Could you check a few things on this model? Use its own coordinates, in mm. Face numbers are marked on the shaded views. Coordinates: 2 decimals unless noted, no trailing zeros. Write each loop counter-clockwise with the first axis right and the second up, starting at its lowest first coordinate (ties: lowest second). Pieces come first, ordered by that corner, then holes. Notation, with made-up numbers: M 78,6.5 L 87,6.5 A34 cw 87,44.5 Z; hole C -21,64.5 d7. An arc over 180 degrees is marked long. Answer as CSV lines item,"result". Start each with the question number.
Item 1: Suppose I cut it at D-D, the plane z = -12.25. Write out the boundary of the cut face in (x, y).
Item 2: Suppose I cut it at B-B, the plane z = -6. Write out the boundary of the cut face in (x, y).
Item 3: If I drill on line 1 along X through (y, z) = (5.5, -7.5); line 2 along X through (y, z) = (22.5, -9); line 3 along Z through (x, y) = (-32, 19), over which ranges is the centre line in solid material (lowest first)? Write a range as [from, to].
Item 4: Suppose I cut it at A-A, the plane y = 7. Write out the boundary of the cut face in (x, z).
Item 5: Suppose I cut it at C-C, the plane x = 12.75. Write out the boundary of the cut face in (y, z), and give its area (3 significant figures).
Item 6: We'd pull the mould along X, two halves only. Please class the marked faces 1, 2, 3 and 4: +X half, -X half, draft (parallel to the pull), parting line (faces both ways), or undercut.
Item 7: I'm going to push flat-ended pins straight in: P1, Ø8, axis at x = 14, y = 15.5, coming from the +Z side; P2, Ø5, axis at x = 10.5, y = 25.5, coming from the -Z side. Where does each tip first touch, or does it pass through?
```python
from build123d import *

# Parameters (mm, degrees)
BOSS_EXTRUDE1_DEPTH = 42
FILLET1_R           = 4
SKETCH2_R           = 4
CUT_EXTRUDE1_DEPTH  = 42
SKETCH3_R           = 2
CUT_EXTRUDE2_DEPTH  = 42


with BuildPart() as part:
    # Sketch1 → Boss-Extrude1 (new body)
    with BuildSketch(Plane(origin=(0, 0, 0), x_dir=(1, 0, 0), z_dir=(0, 1, 0))):
        with BuildLine():
            Line((-37.647058824, 19.411764706), (-42.352941176, 10.588235294))
            ThreePointArc((-42.352941176, 10.588235294), (0, 0), (42.352941176, 10.588235294))
            Line((42.352941176, 10.588235294), (37.647058824, 19.411764706))
            ThreePointArc((37.647058824, 19.411764706), (0, 10), (-37.647058824, 19.411764706))
        make_face()
    extrude(amount=BOSS_EXTRUDE1_DEPTH)

    # Fillet1
    fillet1_edges = [part.edges().sort_by_distance(p)[0] for p in [
        (37.647058824, 21, -19.411764706),
        (42.352941176, 21, -10.588235294),
        (-42.352941176, 21, -10.588235294),
        (-37.647058824, 21, -19.411764706),
    ]]
    fillet(fillet1_edges, radius=FILLET1_R)

    # Sketch2 → Cut-Extrude1 (cut)
    with BuildSketch(Plane(origin=(0, 42, 0), x_dir=(1, 0, 0), z_dir=(0, 1, 0))):
        with Locations(Location((-34, 12.2, 0), (0, 0, 270))):
            Circle(SKETCH2_R)
        with Locations(Location((34, 12.2, 0), (0, 0, 270))):
            Circle(SKETCH2_R)
    extrude(amount=-CUT_EXTRUDE1_DEPTH, mode=Mode.SUBTRACT)

    # Sketch3 → Cut-Extrude2 (cut)
    with BuildSketch(Plane(origin=(0, 42, 0), x_dir=(1, 0, 0), z_dir=(0, 1, 0))):
        with Locations(Location((-12.75, 6, 0), (0, 0, 270))):
            Circle(SKETCH3_R)
        with Locations(Location((12.75, 6, 0), (0, 0, 270))):
            Circle(SKETCH3_R)
    extrude(amount=-CUT_EXTRUDE2_DEPTH, mode=Mode.SUBTRACT)


solid = part.part
```
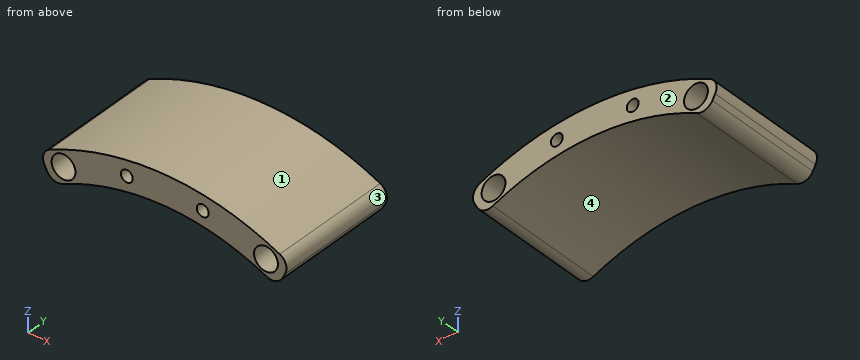
Ans:
1,outline,"M -40.9,0 L -38,0 L -38,42 L -40.9,42 Z; M -30,0 L -18.84,0 L -18.84,42 L -30,42 Z; M 18.84,0 L 30,0 L 30,42 L 18.84,42 Z; M 38,0 L 40.9,0 L 40.9,42 L 38,42 Z"
2,outline,"M -32.31,0 L -14.75,0 L -14.75,42 L -32.31,42 Z; M -10.75,0 L 10.75,0 L 10.75,42 L -10.75,42 Z; M 14.75,0 L 32.31,0 L 32.31,42 L 14.75,42 Z"
3,line 1,"x = [-35.97, -14.07], [-11.43, 11.43], [14.07, 35.97]"
3,line 2,"x = [-39.13, -36.4], [-31.6, 31.6], [36.4, 39.13]"
3,line 3,"z = [-16.68, -15.66], [-8.74, -5.88]"
4,outline,"M -40.43,-14.2 L -39.48,-15.97 A4 ccw -34.24,-17.7 A80 cw 34.24,-17.7 A4 ccw 39.48,-15.97 L 40.43,-14.2 A4 ccw 38.61,-8.7 A90 ccw -38.61,-8.7 A4 ccw Z; hole C -34,-12.2 d8; hole C -12.75,-6 d4; hole C 12.75,-6 d4; hole C 34,-12.2 d8"
5,outline,"M 0,-11.02 L 42,-11.02 L 42,-8 L 0,-8 Z; M 0,-4 L 42,-4 L 42,-0.91 L 0,-0.91 Z"
5,area,"257 mm^2"
6,face 1,"parting line"
6,face 2,"draft"
6,face 3,"+X half"
6,face 4,"undercut"
7,P1,"stops at z = -0.56"
7,P2,"stops at z = -11.06"
